CAD build for the part. Positions are in the model's coordinates, mm. A direction names the side the tool comes from. Give positions to 0.01 mm unless a question says otherwise; leave off trailing zeros. Order: outer loops, then holes, each group sorted by start corner. A loop starts at its lowest first (then second) coordinate and runs counter-clockwise, first axis right, second up.
from build123d import *

# Parameters (mm, degrees)
SKETCH_1_W          = 69.8
SKETCH_1_H          = 31
EXTRUDE_1_DEPTH     = 16.4
SKETCH_2_W          = 9.3
SKETCH_2_H          = 9.85
CUT_EXTRUDE_1_DEPTH = 1
SKETCH_3_W          = 9.3
SKETCH_3_H          = 9.85
CUT_EXTRUDE_2_DEPTH = 13.71
CUT_EXTRUDE_3_DEPTH = 2
HOLE_WIZARD_M3_1_D  = 3.4
SKETCH_8_W          = 0.75
SKETCH_8_H          = 11.3
CUT_EXTRUDE_5_DEPTH = 13.71
SKETCH_9_R          = 0.437276748
EXTRUDE_3_DEPTH     = 2
FILLET_1_R          = 3
FILLET_2_R          = 1


with BuildPart() as part:
    # 草图1 → 凸台-拉伸1 (new body)
    with BuildSketch(Plane.XY):
        Rectangle(SKETCH_1_W, SKETCH_1_H)
    extrude(amount=EXTRUDE_1_DEPTH)

    # 草图2 → 切除-拉伸1 (cut)
    with BuildSketch(Plane(origin=(0, 0, 0), x_dir=(-1, 0, 0), z_dir=(0, 0, -1))):
        with Locations((-30.25, 10.575)):
            Rectangle(SKETCH_2_W, SKETCH_2_H)
        with Locations((-30.25, -10.575)):
            Rectangle(SKETCH_2_W, SKETCH_2_H)
        with Locations((30.25, -10.575)):
            Rectangle(SKETCH_2_W, SKETCH_2_H)
        with Locations((30.25, 10.575)):
            Rectangle(SKETCH_2_W, SKETCH_2_H)
    extrude(amount=-CUT_EXTRUDE_1_DEPTH, mode=Mode.SUBTRACT)

    # 草图3 → 切除-拉伸2 (cut)
    with BuildSketch(Plane.XY.offset(16.4)):
        with Locations((30.25, -10.575)):
            Rectangle(SKETCH_3_W, SKETCH_3_H)
        with Locations((-30.25, -10.575)):
            Rectangle(SKETCH_3_W, SKETCH_3_H)
        with Locations((30.25, 10.575)):
            Rectangle(SKETCH_3_W, SKETCH_3_H)
        with Locations((-30.25, 10.575)):
            Rectangle(SKETCH_3_W, SKETCH_3_H)
    extrude(amount=-CUT_EXTRUDE_2_DEPTH, mode=Mode.SUBTRACT)

    # 草图4 → 切除-拉伸3 (cut)
    with BuildSketch(Plane(origin=(0, 0, 0), x_dir=(-1, 0, 0), z_dir=(0, 0, -1))):
        with BuildLine():
            Line((-2.1, 13.6), (9, 13.6))
            ThreePointArc((9, 13.6), (22.6, 0), (9, -13.6))
            Line((9, -13.6), (-2.1, -13.6))
            ThreePointArc((-2.1, -13.6), (-15.7, 0), (-2.1, 13.6))
        make_face()
    extrude(amount=-CUT_EXTRUDE_3_DEPTH, mode=Mode.SUBTRACT)

    # M3 间隙孔1 (through all)
    with Locations(Plane(origin=(0, 0, 1), x_dir=(-1, 0, 0), z_dir=(0, 0, -1))):
        with Locations((31.75, 12), (31.75, -12), (-31.75, -12), (-31.75, 12)):
            Hole(HOLE_WIZARD_M3_1_D / 2)

    # 草图8 → 切除-拉伸5 (cut)
    with BuildSketch(Plane.XY.offset(16.4)):
        with Locations((-34.525, 0)):
            Rectangle(SKETCH_8_W, SKETCH_8_H)
        with Locations((34.525, 0)):
            Rectangle(SKETCH_8_W, SKETCH_8_H)
    extrude(amount=-CUT_EXTRUDE_5_DEPTH, mode=Mode.SUBTRACT)

    # 草图9 → 凸台-拉伸3 (add)
    with BuildSketch(Plane.ZY.offset(34.15)):
        with Locations(Location((6.232254634, 0, 0), (0, 0, 180))):
            Circle(SKETCH_9_R)
        with Locations(Location((7.500357203, 0, 0), (0, 0, 180))):
            Circle(SKETCH_9_R)
    extrude(amount=EXTRUDE_3_DEPTH)

    # 圆角1
    # the kernel refuses this fillet: 3 mm, written as the material it adds along each edge
    with BuildSketch(Plane(origin=(-9, -13.6, 2), x_dir=(0, 0, -1), z_dir=(1, 0, 0)), Plane(origin=(2.1, 13.6, 2), x_dir=(0, 0, -1), z_dir=(-1, 0, 0))) as fillet_1_piece_1:
        with BuildLine():
            CenterArc((3, 2.828427125), FILLET_1_R, 180, 70.528779366)
            Line((0, 2.828427125), (-0.06, 2.828427125))
            Line((-0.06, 2.828427125), (-0.06, 0))
            Line((-0.06, 0), (0, -0.06))
            ThreePointArc((0, -0.06), (1, -0.06), (1.98, -0.056568542))
            Line((1.98, -0.056568542), (2, 0))
        make_face()
    extrude(amount=11.1)
    with BuildSketch(Plane(origin=(2.1, 0, 2), x_dir=(0, -1, 0), z_dir=(-1, 0, 0))) as fillet_1_piece_2:
        with BuildLine():
            CenterArc((10.771572875, -3), FILLET_1_R, 19.471220634, 70.528779366)
            Line((10.771572875, 0), (10.771572875, 0.06))
            Line((10.771572875, 0.06), (13.6, 0.06))
            Line((13.6, 0.06), (13.66, 0))
            ThreePointArc((13.66, 0), (13.66, -1), (13.656568542, -1.98))
            Line((13.656568542, -1.98), (13.6, -2))
        make_face()
    revolve(axis=Axis((2.1, 0, 2), (0, 0, 1)), revolution_arc=180)
    with BuildSketch(Plane(origin=(-9, 0, 2), x_dir=(0, 1, 0), z_dir=(1, 0, 0))) as fillet_1_piece_3:
        with BuildLine():
            CenterArc((10.771572875, -3), FILLET_1_R, 19.471220634, 70.528779366)
            Line((10.771572875, 0), (10.771572875, 0.06))
            Line((10.771572875, 0.06), (13.6, 0.06))
            Line((13.6, 0.06), (13.66, 0))
            ThreePointArc((13.66, 0), (13.66, -1), (13.656568542, -1.98))
            Line((13.656568542, -1.98), (13.6, -2))
        make_face()
    revolve(axis=Axis((-9, 0, 2), (0, 0, 1)), revolution_arc=180)
    with BuildSketch(Plane(origin=(-25.6, -5.65, 0), x_dir=(0, -1, 0), z_dir=(0, 0, 1)), Plane(origin=(-25.6, 5.65, 0), x_dir=(-1, 0, 0), z_dir=(0, 0, 1))) as fillet_1_piece_4:
        with BuildLine():
            CenterArc((FILLET_1_R, -FILLET_1_R), FILLET_1_R, 90, 90)
            Line((0, -FILLET_1_R), (-FILLET_1_R * 0.02, -FILLET_1_R))
            Line((-FILLET_1_R * 0.02, -FILLET_1_R), (-FILLET_1_R * 0.02, FILLET_1_R * 0.02))
            Line((-FILLET_1_R * 0.02, FILLET_1_R * 0.02), (FILLET_1_R, FILLET_1_R * 0.02))
            Line((FILLET_1_R, FILLET_1_R * 0.02), (FILLET_1_R, 0))
        make_face()
    extrude(amount=8.5)
    with BuildSketch(Plane(origin=(25.6, -5.65, 0), x_dir=(0, -1, 0), z_dir=(0, 0, 1)), Plane(origin=(25.6, 5.65, 0), x_dir=(1, 0, 0), z_dir=(0, 0, 1))) as fillet_1_piece_5:
        with BuildLine():
            CenterArc((FILLET_1_R, FILLET_1_R), FILLET_1_R, 180, 90)
            Line((0, FILLET_1_R), (-FILLET_1_R * 0.02, FILLET_1_R))
            Line((-FILLET_1_R * 0.02, FILLET_1_R), (-FILLET_1_R * 0.02, -FILLET_1_R * 0.02))
            Line((-FILLET_1_R * 0.02, -FILLET_1_R * 0.02), (FILLET_1_R, -FILLET_1_R * 0.02))
            Line((FILLET_1_R, -FILLET_1_R * 0.02), (FILLET_1_R, 0))
        make_face()
    extrude(amount=8.5)
    with BuildSketch(Plane(origin=(-25.6, 5.65, 16.4), x_dir=(-1, 0, 0), z_dir=(0, 0, -1))) as fillet_1_piece_6_section:
        with BuildLine():
            CenterArc((FILLET_1_R, FILLET_1_R), FILLET_1_R, 180, 90)
            Line((0, FILLET_1_R), (-FILLET_1_R * 0.02, FILLET_1_R))
            Line((-FILLET_1_R * 0.02, FILLET_1_R), (-FILLET_1_R * 0.02, -FILLET_1_R * 0.02))
            Line((-FILLET_1_R * 0.02, -FILLET_1_R * 0.02), (FILLET_1_R, -FILLET_1_R * 0.02))
            Line((FILLET_1_R, -FILLET_1_R * 0.02), (FILLET_1_R, 0))
        make_face()
    fillet_1_piece_6 = extrude(amount=21.21, mode=Mode.PRIVATE)
    fillet_1_piece_6 = split(fillet_1_piece_6, bisect_by=Plane(origin=(-26.279185343, 6.329185343, 0), z_dir=(0, 0, 1)), keep=Keep.TOP, mode=Mode.PRIVATE)
    add(fillet_1_piece_6)
    with BuildSketch(Plane(origin=(25.6, 5.65, 16.4), x_dir=(1, 0, 0), z_dir=(0, 0, -1))) as fillet_1_piece_7_section:
        with BuildLine():
            CenterArc((FILLET_1_R, -FILLET_1_R), FILLET_1_R, 90, 90)
            Line((0, -FILLET_1_R), (-FILLET_1_R * 0.02, -FILLET_1_R))
            Line((-FILLET_1_R * 0.02, -FILLET_1_R), (-FILLET_1_R * 0.02, FILLET_1_R * 0.02))
            Line((-FILLET_1_R * 0.02, FILLET_1_R * 0.02), (FILLET_1_R, FILLET_1_R * 0.02))
            Line((FILLET_1_R, FILLET_1_R * 0.02), (FILLET_1_R, 0))
        make_face()
    fillet_1_piece_7 = extrude(amount=21.21, mode=Mode.PRIVATE)
    fillet_1_piece_7 = split(fillet_1_piece_7, bisect_by=Plane(origin=(26.279185343, 6.329185343, 0), z_dir=(0, 0, 1)), keep=Keep.TOP, mode=Mode.PRIVATE)
    add(fillet_1_piece_7)
    with BuildSketch(Plane(origin=(25.6, -5.65, 16.4), x_dir=(0, -1, 0), z_dir=(0, 0, -1))) as fillet_1_piece_8_section:
        with BuildLine():
            CenterArc((FILLET_1_R, -FILLET_1_R), FILLET_1_R, 90, 90)
            Line((0, -FILLET_1_R), (-FILLET_1_R * 0.02, -FILLET_1_R))
            Line((-FILLET_1_R * 0.02, -FILLET_1_R), (-FILLET_1_R * 0.02, FILLET_1_R * 0.02))
            Line((-FILLET_1_R * 0.02, FILLET_1_R * 0.02), (FILLET_1_R, FILLET_1_R * 0.02))
            Line((FILLET_1_R, FILLET_1_R * 0.02), (FILLET_1_R, 0))
        make_face()
    fillet_1_piece_8 = extrude(amount=21.21, mode=Mode.PRIVATE)
    fillet_1_piece_8 = split(fillet_1_piece_8, bisect_by=Plane(origin=(26.279185343, -6.329185343, 0), z_dir=(0, 0, 1)), keep=Keep.TOP, mode=Mode.PRIVATE)
    add(fillet_1_piece_8)
    with BuildSketch(Plane(origin=(-25.6, -5.65, 16.4), x_dir=(0, -1, 0), z_dir=(0, 0, -1))) as fillet_1_piece_9_section:
        with BuildLine():
            CenterArc((FILLET_1_R, FILLET_1_R), FILLET_1_R, 180, 90)
            Line((0, FILLET_1_R), (-FILLET_1_R * 0.02, FILLET_1_R))
            Line((-FILLET_1_R * 0.02, FILLET_1_R), (-FILLET_1_R * 0.02, -FILLET_1_R * 0.02))
            Line((-FILLET_1_R * 0.02, -FILLET_1_R * 0.02), (FILLET_1_R, -FILLET_1_R * 0.02))
            Line((FILLET_1_R, -FILLET_1_R * 0.02), (FILLET_1_R, 0))
        make_face()
    fillet_1_piece_9 = extrude(amount=21.21, mode=Mode.PRIVATE)
    fillet_1_piece_9 = split(fillet_1_piece_9, bisect_by=Plane(origin=(-26.279185343, -6.329185343, 0), z_dir=(0, 0, 1)), keep=Keep.TOP, mode=Mode.PRIVATE)
    add(fillet_1_piece_9)

    # 圆角2
    fillet_2_edges = [part.edges().sort_by_distance(p)[0] for p in [
        (-25.6, 15.5, 9.545),
        (-34.15, -5.65, 9.545),
        (-34.15, 5.65, 9.545),
        (34.15, 5.65, 9.545),
        (34.15, -5.65, 9.545),
        (34.9, -15.5, 1.845),
        (25.6, -15.5, 9.545),
        (-34.9, 15.5, 1.845),
        (34.9, 15.5, 1.845),
        (-34.9, -15.5, 1.845),
        (25.6, 15.5, 9.545),
        (-25.6, -15.5, 9.545),
    ]]
    fillet(fillet_2_edges, radius=FILLET_2_R)


solid = part.part
1. 3-axis set-ups, long thin cutter, end or side, ignore diameter. For faces 1 (the flat face through (-25.6, -12, 10)), 2 (the flat face through (-31, 5.65, 10)), 3 (the flat face through (31, 5.65, 10)): which of +Z, -Z, +X, -X, +Y, -Y reach the whole face in a straight line?
2. Saw through at D-D on y = -12. State how many separate pieces and enclosed holes the cut face has, plus the area to 3 significant figures.
3. Saw through at B-B on z = 12.5. Give the cut face in (x, y), plus the area to 3 significant figures.
4. Wall check: line 1 (Y direction, x = 31.75, z = 1.9); line 2 (Y direction, x = -30, z = 11.75); line 3 (X direction, y = 13.5, z = 14.5). Give the ranges that are in metal, low to high.
5. Saw through at A-A on x = -31.75. Give the cut face in (y, z).
6. Saw through at C-C on x = -7. Give the cut face in (y, z).
7. Pin check, flat tips, straight feed: P1, Ø1, axis at x = 19, y = -2.5, coming from the -Z side; P2, Ø3, axis at y = -7.5, z = 3.5, coming from the -X side; P3, Ø1, axis at x = 27, y = -10.5, coming from the +Z side; P4, Ø4, axis at y = 6, z = 11, coming from the -X side. Stop position of each tip, or through.
Reported:
1. face 1: +Z, -X, -Y
1. face 2: +Z, -X, +Y
1. face 3: +Z, +X, +Y
2. separate pieces: 3
2. enclosed holes: 0
2. area: 823 mm2
3. outline: (-34.15, -4.65) arc R1 ccw to (-33.15, -5.65) - (-28.6, -5.65) arc R3 cw to (-25.6, -8.65) - (-25.6, -14.5) arc R1 ccw to (-24.6, -15.5) - (24.6, -15.5) arc R1 ccw to (25.6, -14.5) - (25.6, -8.65) arc R3 cw to (28.6, -5.65) - (33.15, -5.65) arc R1 ccw to (34.15, -4.65) - (34.15, 4.65) arc R1 ccw to (33.15, 5.65) - (28.6, 5.65) arc R3 cw to (25.6, 8.65) - (25.6, 14.5) arc R1 ccw to (24.6, 15.5) - (-24.6, 15.5) arc R1 ccw to (-25.6, 14.5) - (-25.6, 8.65) arc R3 cw to (-28.6, 5.65) - (-33.15, 5.65) arc R1 ccw to (-34.15, 4.65) - close
3. area: 1,790 mm2
4. line 1: y = -15.5 to -13.7, -10.3 to 10.3, 13.7 to 15.5
4. line 2: y = -5.65 to 5.65
4. line 3: x = -25.6 to 25.6
5. outline: (-15.5, 1) - (-13.7, 1) - (-13.7, 2.69) - (-15.5, 2.69) - close; (-10.3, 1) - (-5.65, 1) - (-5.65, 0) - (5.65, 0) - (5.65, 1) - (10.3, 1) - (10.3, 2.69) - (5.65, 2.69) - (5.65, 16.4) - (-5.65, 16.4) - (-5.65, 2.69) - (-10.3, 2.69) - close; (13.7, 1) - (15.5, 1) - (15.5, 2.69) - (13.7, 2.69) - close
6. outline: (-15.5, 0) - (-13.6, 0) arc R3 cw to (-10.77, 2) - (10.77, 2) arc R3 cw to (13.6, 0) - (15.5, 0) - (15.5, 16.4) - (-15.5, 16.4) - close
7. P1: stops at z = 0
7. P2: stops at x = -34.9
7. P3: stops at z = 2.69
7. P4: stops at x = -34.15
